from build123d import *

# Parameters (mm, degrees)
SKETCH1_W                 = 5.5
SKETCH1_H                 = 12.3
BOSS_EXTRUDE1_DEPTH       = 4.8
SKETCH2_W                 = 2.3
SKETCH2_H                 = 9.3
CUT_EXTRUDE1_DEPTH        = 6.5
SKETCH3_W                 = 2.5
SKETCH3_H                 = 5.1
BOSS_EXTRUDE2_DEPTH       = 22.5
SKETCH4_W                 = 5.5
SKETCH4_H                 = 2.5
BOSS_EXTRUDE3_DEPTH       = 7.2
SKETCH5_W                 = 5.5
SKETCH5_H                 = 3
BOSS_EXTRUDE4_DEPTH       = 2.3
F_2_CLEARANCE_HOLE1_D     = 2.6
F_2_CLEARANCE_HOLE1_DEPTH = 4.8
F_1_CLEARANCE_HOLE1_D     = 2.05
F_1_CLEARANCE_HOLE1_DEPTH = 4
F_1_CLEARANCE_HOLE1_TIP   = 0.615882135
CHAMFER1_SIZE             = 0.3
CHAMFER2_SIZE             = 0.2
FILLET1_R                 = 1.5


with BuildPart() as part:
    # Sketch1 → Boss-Extrude1 (new body)
    with BuildSketch(Plane(origin=(0, 0, -2.5), x_dir=(-1, 0, 0), z_dir=(0, 0, -1))):
        with Locations((-11.25, 6.15)):
            Rectangle(SKETCH1_W, SKETCH1_H)
    extrude(amount=-BOSS_EXTRUDE1_DEPTH)

    # Sketch2 → Cut-Extrude1 (cut, through all)
    with BuildSketch(Plane.ZY.offset(-8.5)):
        with Locations((1.15, 7.65)):
            Rectangle(SKETCH2_W, SKETCH2_H)
    extrude(amount=-CUT_EXTRUDE1_DEPTH, mode=Mode.SUBTRACT)

    # Sketch3 → Boss-Extrude2 (add)
    with BuildSketch(Plane.ZY.offset(-8.5)):
        with Locations((-1.25, 9.75)):
            Rectangle(SKETCH3_W, SKETCH3_H)
    extrude(amount=BOSS_EXTRUDE2_DEPTH)

    # Sketch4 → Boss-Extrude3 (add)
    with BuildSketch(Plane.XZ.offset(-7.2)):
        with Locations((-11.25, -1.25)):
            Rectangle(SKETCH4_W, SKETCH4_H)
    extrude(amount=BOSS_EXTRUDE3_DEPTH)

    # Sketch5 → Boss-Extrude4 (add)
    with BuildSketch(Plane.XY):
        with Locations((-11.25, 1.5)):
            Rectangle(SKETCH5_W, SKETCH5_H)
    extrude(amount=BOSS_EXTRUDE4_DEPTH)

    # #2 Clearance Hole1
    with Locations(Plane(origin=(0, 0, -2.5), x_dir=(-1, 0, 0), z_dir=(0, 0, -1))):
        with Locations((11, 9.7), (-11, 9.7)):
            Hole(F_2_CLEARANCE_HOLE1_D / 2, depth=F_2_CLEARANCE_HOLE1_DEPTH)

    # #1 Clearance Hole1
    with Locations(Plane(origin=(0, 0, 0), x_dir=(-1, 0, 0), z_dir=(0, -1, 0))):
        with Locations((-11, 0.3), (11, 0.3)):
            Hole(F_1_CLEARANCE_HOLE1_D / 2, depth=F_1_CLEARANCE_HOLE1_DEPTH)
            with Locations((0, 0, -(F_1_CLEARANCE_HOLE1_DEPTH + F_1_CLEARANCE_HOLE1_TIP / 2))):  # 118° drill point
                Cone(0, F_1_CLEARANCE_HOLE1_D / 2, F_1_CLEARANCE_HOLE1_TIP, mode=Mode.SUBTRACT)

    # Chamfer1
    chamfer1_edges = [part.edges().sort_by_distance(p)[0] for p in [
        (11.25, 3, 2.3),
        (0, 12.3, 0),
        (11.25, 0, 2.3),
        (-11.25, 0, -2.5),
        (0, 12.3, -2.5),
        (-11.25, 0, 2.3),
        (11.25, 0, -2.5),
        (-11.25, 3, 2.3),
        (9.7, 9.7, -2.5),
        (-12.025, 0, -0.3),
        (9.975, 0, -0.3),
    ]]
    chamfer(chamfer1_edges, length=CHAMFER1_SIZE)

    # Chamfer2
    chamfer2_edges = [part.edges().sort_by_distance(p)[0] for p in [
        (-12.3, 9.7, -2.5),
    ]]
    chamfer(chamfer2_edges, length=CHAMFER2_SIZE)

    # Fillet1
    fillet1_edges = [part.edges().sort_by_distance(p)[0] for p in [
        (8.5, 7.2, -1.25),
        (-8.5, 7.2, -1.25),
    ]]
    fillet(fillet1_edges, radius=FILLET1_R)


solid = part.part
Work out the finished part from the listing and answer in its coordinate system (mm). A direction names the side the tool comes from. Round coordinates to 2 decimals unless told otherwise and drop trailing zeros. Order: outer loops, then holes, each group sorted by start corner. A loop starts at its lowest first (then second) coordinate and runs counter-clockwise, first axis right, second up. Notation, with made-up numbers: M 70,74.25 L 125,74.25 A22 cw 125,98.25 Z; hole C 32.25,-9 d3. An arc over 180 degrees is marked long. Put each result on its own line as item: value. Start each with the question number.
Q1. Section D-D, the plane z = 0.3 is taken. Give the number of separate pieces and of enclosed holes in the cut face, and give its area (3 significant figures).
Q2. Section A-A, the plane y = 9.7 is taken. Write down the section's boundary in (x, z).
Q3. Section B-B, the plane y = 3.25 is taken. Write down the section's boundary in (x, z) (3 decimals), and give its area (3 significant figures).
Q4. A tool of negligible diameter and unlimited length cuts with its end or side. For faces 1 (the cylindrical face through (-10.4, 8.547, -1.134)), 2 (the cylindrical face through (-11.133, 2.176, -1.316)), 3 (the flat face through (-11, 3, 1)), 4 (the flat face through (8.5, 2, -1)), 5 (the flat face through (-11, 2, 2.3)), from which of +Z, -Z, +X, -X, +Y, -Y can it reach the whole face along a straight path? Write none if from no direction.
Q5. Section C-C, the plane x = -9 is taken. Write down the section's boundary in (y, z).
Q6. For a pull along Z with two mould halves and no side action, classify faces 6 (the flat face through (0, 9, 0)), 7 (the flat face through (0, 12.3, -1)), 8 (the conical face through (-10.96, 4.44, -0.59)) as pulls with the +Z half, pulls with the -Z half, needs draft (parallel to the pull), parting line crosses it, or undercut.
Q7. Straight lines are drawn through the part: L1, parallel to X at y = 1.75, z = -0.3 (3 decimals); L2, parallel to Z at x = 11, y = 2.1 (3 decimals); L3, parallel to Z at x = -5.75, y = 8.75. For each, find the intervals that lie inside material, in ascending order. Write a range as [from, to].
Q8. Flat-ended cylindrical pins translate along their axes: pin 1 (5 mm diameter, centred on x = 7.5, y = 3.5, fed in from -Z); pin 2 (2.5 mm diameter, centred on x = -2.5, y = 6.5, fed in from +Z); pin 3 (1.5 mm diameter, centred on x = 3.5, z = 0.5, fed in from +Y); pin 4 (1.6 mm diameter, centred on x = 11, z = -0.3, fed in from -Y). Find the tip coordinate at first contact, or state that the pin passes through.
Findings below:
1. separate pieces: 4
1. enclosed holes: 0
1. area: 22.8 mm^2
2. outline: M -14,-2.5 L -12.5,-2.5 L -12.3,-2.3 L -12.3,0 L -14,0 Z; M -9.7,-2.3 L -9.5,-2.5 L 9.4,-2.5 L 9.7,-2.2 L 9.7,0 L -9.7,0 Z; M 12.3,-2.2 L 12.6,-2.5 L 14,-2.5 L 14,0 L 12.3,0 Z
3. outline: M -14,-2.5 L -8.5,-2.5 L -8.5,0 L -10.02,0 A1.025 cw long -11.98,0 L -14,0 Z; M 8.5,-2.5 L 14,-2.5 L 14,0 L 11.98,0 A1.025 cw long 10.02,0 L 8.5,0 Z
3. area: 23.0 mm^2
4. face 1: +Z, -Z
4. face 2: -Y
4. face 3: +Z, +X, -X, +Y
4. face 4: +Z, -Z, -Y
4. face 5: +Z, +X, -X, +Y, -Y
5. outline: M 0,-2.2 L 0.3,-2.5 L 12,-2.5 L 12.3,-2.2 L 12.3,-0.3 L 12,0 L 3,0 L 3,2 L 2.7,2.3 L 0.3,2.3 L 0,2 Z
6. face 6: pulls with the +Z half
6. face 7: needs draft
6. face 8: undercut
7. L1: x = [-14, -12.025], [-9.975, -8.5], [8.5, 9.975], [12.025, 14]
7. L2: z = [-2.5, -1.325], [0.725, 2.3]
7. L3: z = [-2.5, 0]
8. pin 1: stops at z = -2.5
8. pin 2: stops at z = 0
8. pin 3: stops at y = 12.25
8. pin 4: stops at y = 4.14
